```python
from build123d import *

# Parameters (mm, degrees)
BOSS_EXTRUDE1_DEPTH = 6.35
SKETCH2_R           = 3.175
CUT_EXTRUDE1_DEPTH  = 26.4
SKETCH3_R           = 3.175
CUT_EXTRUDE2_DEPTH  = 20.05


with BuildPart() as part:
    # Sketch1 → Boss-Extrude1 (new body, symmetric)
    with BuildSketch(Plane.XY):
        Polygon((-12.7, 38.1), (-12.7, 15.875), (-6.35, 15.875), (-6.35, 0), (6.35, 0), (6.35, 15.875), (12.7, 15.875), (12.7, 38.1), (7.9375, 38.1), (7.9375, 22.225), (-7.9375, 22.225), (-7.9375, 38.1), align=None)
    extrude(amount=BOSS_EXTRUDE1_DEPTH, both=True)

    # Sketch2 → Cut-Extrude1 (cut, through all)
    with BuildSketch(Plane(origin=(12.7, 0, 0), x_dir=(0, 0, -1), z_dir=(1, 0, 0))):
        with Locations((0, 31.75)):
            Circle(SKETCH2_R)
    extrude(amount=-CUT_EXTRUDE1_DEPTH, mode=Mode.SUBTRACT)

    # Sketch3 → Cut-Extrude2 (cut, through all)
    with BuildSketch(Plane(origin=(6.35, 0, 0), x_dir=(0, 0, -1), z_dir=(1, 0, 0))):
        with Locations((0, 6.35)):
            Circle(SKETCH3_R)
    extrude(amount=-CUT_EXTRUDE2_DEPTH, mode=Mode.SUBTRACT)


solid = part.part
```
For this review, take the finished solid that the model builds, in its own axes (mm). A direction names the side the tool comes from. Coordinates: 2 decimals unless noted, no trailing zeros. Write each loop counter-clockwise with the first axis right and the second up, starting at its lowest first coordinate (ties: lowest second). Pieces come first, ordered by that corner, then holes.
(1) For pin 1 Ø1.5 at (x, z) = (6.5, -2.5) entering from +Y (3 decimals); pin 2 Ø6.5 at (y, z) = (7, -2.5) entering from +X; pin 3 Ø1.9 at (x, z) = (8.5, 1.5) entering from -Y (3 decimals), all flat-tipped, find the tip position at first contact; note any pin that passes through.
(2) Tool access review of faces 1 (the face through (0, 22.225, 0)), 2 (the face through (-6.35, 10, 0)), 3 (the face through (9, 15.875, 0)), 4 (the face through (12.7, 27, 0)): name each direction out of +Z, -Z, +X, -X, +Y, -Y from which nothing blocks a thin tool from reaching the whole face with its end or side.
(3) The part is to be moulded in two halves that separate along X. For faces 5 (the face through (6.35, 10, 0)), 6 (the face through (-10, 15.875, 0)), 7 (the face through (7.938, 29, 2)), say which applies: +X half, -X half, draft (parallel to the pull), parting line (faces both ways), or undercut.
(4) Wall thickness on probe 1 along Y at (x, z) = (-9, 0) (3 decimals); probe 2 along Y at (x, z) = (0, 0) (3 decimals); probe 3 along X at (y, z) = (2.5, 2.75): over which ranges is each line inside the solid? List them lowest first.
(5) Add section B-B on z = 0. Count the separate pieces of the cut face and the enclosed holes in it, then the cut area to 3 significant figures.
(6) Add section A-A on y = 6.35. Give the boundary of the cut face in (x, z) (3 decimals).
Answer sheet:
1. pin 1: stops at y = 22.225
1. pin 2: stops at x = 6.35
1. pin 3: stops at y = 15.875
2. face 1: +Z, -Z, +Y
2. face 2: +Z, -Z, -X, -Y
2. face 3: +Z, -Z, +X, -Y
2. face 4: +Z, -Z, +X, +Y, -Y
3. face 5: +X half
3. face 6: draft
3. face 7: undercut
4. probe 1: y = 15.875 to 28.575, 34.925 to 38.1
4. probe 2: y = 0 to 3.175, 9.525 to 22.225
4. probe 3: x = -6.35 to 6.35
5. separate pieces: 4
5. enclosed holes: 0
5. area: 373 mm2
6. outline: (-6.35, -6.35) - (6.35, -6.35) - (6.35, -3.175) - (-6.35, -3.175) - close; (-6.35, 3.175) - (6.35, 3.175) - (6.35, 6.35) - (-6.35, 6.35) - close
